```python
from build123d import *

# Parameters (mm, degrees)
SKETCH1_R           = 5.8
SKETCH1_R_2         = 4.05
BOSS_EXTRUDE1_DEPTH = 6.8875
CUT_EXTRUDE1_START  = -5.1375
CUT_EXTRUDE1_DEPTH  = 10.274999888
CUT_EXTRUDE2_START  = 6.8875
SKETCH1_5_R         = 4.05
CUT_EXTRUDE2_DEPTH  = 4.8
CUT_EXTRUDE3_DEPTH  = 28.681774239


with BuildPart() as part:
    # Sketch1 → Boss-Extrude1 (new, symmetric)
    with BuildSketch(Plane(origin=(0, 0, 0), x_dir=(1, 0, 0), z_dir=(0, 1, 0))):
        with BuildLine():
            ThreePointArc((-5.597034746, -1.520921448), (-4.307408497, -7.915763352), (-3.875, -14.425))
            Line((-3.875, -14.425), (-3.875, -19.425))
            ThreePointArc((-3.875, -19.425), (0, -23.3), (3.875, -19.425))
            Line((3.875, -19.425), (3.875, -14.425))
            ThreePointArc((3.875, -14.425), (4.307408497, -7.915763352), (5.597034746, -1.520921448))
            ThreePointArc((5.597034746, -1.520921448), (0, -5.8), (-5.597034746, -1.520921448))
        make_face()
        with BuildLine():
            ThreePointArc((-1.875, -9.425), (0, -7.55), (1.875, -9.425))
            Line((1.875, -9.425), (1.875, -19.425))
            ThreePointArc((1.875, -19.425), (0, -21.3), (-1.875, -19.425))
            Line((-1.875, -19.425), (-1.875, -9.425))
        make_face(mode=Mode.SUBTRACT)
        Circle(SKETCH1_R)
        Circle(SKETCH1_R_2, mode=Mode.SUBTRACT)
        Circle(SKETCH1_R_2)
    extrude(amount=BOSS_EXTRUDE1_DEPTH, both=True)

    # Sketch1<4> → Cut-Extrude1 (cut)
    with BuildSketch(Plane(origin=(0, 0, 0), x_dir=(1, 0, 0), z_dir=(0, 1, 0)).offset(CUT_EXTRUDE1_START)):
        with BuildLine():
            ThreePointArc((-5.597034746, -1.520921448), (-4.307408497, -7.915763352), (-3.875, -14.425))
            Line((-3.875, -14.425), (-3.875, -19.425))
            ThreePointArc((-3.875, -19.425), (0, -23.3), (3.875, -19.425))
            Line((3.875, -19.425), (3.875, -14.425))
            ThreePointArc((3.875, -14.425), (4.307408497, -7.915763352), (5.597034746, -1.520921448))
            ThreePointArc((5.597034746, -1.520921448), (0, -5.8), (-5.597034746, -1.520921448))
        make_face()
        with BuildLine():
            ThreePointArc((-1.875, -9.425), (0, -7.55), (1.875, -9.425))
            Line((1.875, -9.425), (1.875, -19.425))
            ThreePointArc((1.875, -19.425), (0, -21.3), (-1.875, -19.425))
            Line((-1.875, -19.425), (-1.875, -9.425))
        make_face(mode=Mode.SUBTRACT)
    extrude(amount=CUT_EXTRUDE1_DEPTH, mode=Mode.SUBTRACT)

    # Sketch1<5> → Cut-Extrude2 (cut)
    with BuildSketch(Plane(origin=(0, 0, 0), x_dir=(1, 0, 0), z_dir=(0, 1, 0)).offset(CUT_EXTRUDE2_START)):
        with Locations(Location((0, 0, 0), (0, 0, 270))):
            Circle(SKETCH1_5_R)
    extrude(amount=-CUT_EXTRUDE2_DEPTH, mode=Mode.SUBTRACT)

    # Sketch4 → Cut-Extrude3 (cut, through all)
    with BuildSketch(Plane.XZ.offset(6.8875)):
        with BuildLine():
            ThreePointArc((-3.875, 19.425), (0, 22.55), (3.875, 19.425))
            ThreePointArc((3.875, 19.425), (0, 23.3), (-3.875, 19.425))
        make_face()
    extrude(amount=-CUT_EXTRUDE3_DEPTH, mode=Mode.SUBTRACT)


solid = part.part
```
Model file for the job. Use its own axes, mm. A direction names the side the tool comes from. Coordinates: 2 decimals unless noted, no trailing zeros. Order: outer loops, then holes, each group sorted by start corner. A loop starts at its lowest first (then second) coordinate and runs counter-clockwise, first axis right, second up. Notation, with made-up numbers: (34.25, 78) -> (74.25, 78) arc R22 ccw to (74.25, 84) -> close; hole circle Ø7 at (-10, 21). An arc over 180 degrees is marked (long way). Answer as a JSON object with one key per item and string values. Group by question number.
1) Cut at B-B, the plane z = 14.75. Write the cut outline in (x, y) (1 decimal), then the cut area to 3 significant figures.
2) Cut at A-A, the plane x = 0. Write the cut outline in (y, z).
3) Cut at C-C, the plane y = 6. Write the cut outline in (x, z) (3 decimals).
4) Flat gauge pins, fed straight in: pin 1 (3.5 mm diameter, centred on x = -0.5, z = 15, fed in from -Y); pin 2 (2 mm diameter, centred on x = 2.5, y = -2, fed in from +Z); pin 3 (0.9 mm diameter, centred on y = -5.5, z = 17.5, fed in from +X) (3 decimals); pin 4 (0.5 mm diameter, centred on y = 6.5, z = 17.5, fed in from -X) (3 decimals). Where does each tip first touch, or does it go through?
5) Pull direction Z, two halves, no side cores. Call faces 1 (the face through (4.295, -6, 8.006)), 2 (the face through (0, -6.888, 5)), 3 (the face through (0, -6, 21.3)): +Z half, -Z half, draft (parallel to the pull), parting line (faces both ways), or undercut.
6) Drill centre lines: L1, parallel to X at y = 4.5, z = 0; L2, parallel to Y at x = 4, z = 5.25; L3, parallel to Z at x = -1.5, y = -3.75. Where is each one in solid material? Low to high.
7) Which spindle directions (+Z, -Z, +X, -X, +Y, -Y) get a long thin tool onto all of the face, cutting with end or side? Do faces 4 (the face through (-3.875, 6, 17)), 5 (the face through (3.875, -6, 17)), 6 (the face through (-0.04, -6, 7.55)), 7 (the face through (0, 2.088, 0)), 8 (the face through (-0.08, -6.02, 22.55)). Say none if no direction does.
8) Cut at D-D, the plane z = 0. Write the cut outline in (x, y).
Check values:
{
 "1": {"outline": "(-3.9, -6.9) -> (-1.9, -6.9) -> (-1.9, -5.1) -> (-3.9, -5.1) -> close; (-3.9, 5.1) -> (-1.9, 5.1) -> (-1.9, 6.9) -> (-3.9, 6.9) -> close; (1.9, -6.9) -> (3.9, -6.9) -> (3.9, -5.1) -> (1.9, -5.1) -> close; (1.9, 5.1) -> (3.9, 5.1) -> (3.9, 6.9) -> (1.9, 6.9) -> close", "area": "14.0 mm²"},
 "2": {"outline": "(-6.89, -5.8) -> (6.89, -5.8) -> (6.89, -4.05) -> (2.09, -4.05) -> (2.09, 4.05) -> (6.89, 4.05) -> (6.89, 7.55) -> (5.14, 7.55) -> (5.14, 5.8) -> (-5.14, 5.8) -> (-5.14, 7.55) -> (-6.89, 7.55) -> close; (-6.89, 21.3) -> (-5.14, 21.3) -> (-5.14, 22.55) -> (-6.89, 22.55) -> close; (5.14, 21.3) -> (6.89, 21.3) -> (6.89, 22.55) -> (5.14, 22.55) -> close"},
 "3": {"outline": "(-5.597, 1.521) arc R5.8 ccw (long way) to (5.597, 1.521) arc R49.209 cw to (3.875, 14.425) -> (3.875, 19.425) arc R3.965 ccw to (-3.875, 19.425) -> (-3.875, 14.425) arc R49.209 cw to start; hole circle Ø8.1 at (0, 0); hole (-1.875, 9.425) arc R1.875 ccw to (1.875, 9.425) -> (1.875, 19.425) arc R1.875 ccw to (-1.875, 19.425) -> close"},
 "4": {"pin 1": "stops at y = -6.89", "pin 2": "stops at z = 5.6", "pin 3": "stops at x = 3.875", "pin 4": "stops at x = -3.875"},
 "5": {"face 1": "+Z half", "face 2": "draft", "face 3": "undercut"},
 "6": {"L1": "x = -5.8 to -4.05, 4.05 to 5.8", "L2": "y = -6.89 to -5.14, 5.14 to 6.89", "L3": "z = -5.6 to 5.6"},
 "7": {"face 4": "+Z, -X, +Y, -Y", "face 5": "+Z, +X, +Y, -Y", "face 6": "+Y, -Y", "face 7": "+Y", "face 8": "+Z, +Y, -Y"},
 "8": {"outline": "(-5.8, -6.89) -> (5.8, -6.89) -> (5.8, 6.89) -> (4.05, 6.89) -> (4.05, 2.09) -> (-4.05, 2.09) -> (-4.05, 6.89) -> (-5.8, 6.89) -> close"}
}
